The model under review builds one solid part; all positions refer to its coordinate system, in mm. Round coordinates to 2 decimals unless told otherwise and drop trailing zeros. Return JSON: item names as keys, results as strings. Group by question number.
Q1. Consider section A-A (y = 0). Count the separate pieces of the cut face and the enclosed holes in it, and give its area (3 significant figures).
Q2. To check wall thickness, follow line 1 along Y through (x, z) = (0, 0.1) (3 decimals); line 2 along Y through (x, z) = (5.5, 1.3). State the ranges of each line that lie inside material, in increasing order.
Q3. Clearance check with flat-ended pins moving along their axes: pin 1 Ø2 at (y, z) = (1, 1.5) entering from +X; pin 2 Ø1 at (x, z) = (-6, 2.5) entering from +Y; pin 3 Ø2 at (y, z) = (0, 0.5) entering from -X. State where each tip first meets the part, or that it passes through.
from build123d import *

# Parameters (mm, degrees)
SKETCH_1_R      = 16
SKETCH_1_R_2    = 12.5
EXTRUDE_1_DEPTH = 4
EXTRUDE_START   = -2
SKETCH_2_R      = 17
SKETCH_2_R_2    = 16
EXTRUDE_2_DEPTH = 1.1
FILLET_1_R      = 0.1
SKETCH_3_W      = 0.5
SKETCH_3_H      = 1.15


with BuildPart() as part:
    # 草图1 → 凸台-拉伸1 (new body)
    with BuildSketch(Plane.XY):
        Circle(SKETCH_1_R)
        Circle(SKETCH_1_R_2, mode=Mode.SUBTRACT)
    extrude(amount=EXTRUDE_1_DEPTH)

    # 草图2 → 凸台-拉伸2 (add)
    with BuildSketch(Plane.XY.offset(4).offset(EXTRUDE_START)):
        Circle(SKETCH_2_R)
        Circle(SKETCH_2_R_2, mode=Mode.SUBTRACT)
    extrude(amount=EXTRUDE_2_DEPTH)

    # 圆角1
    fillet_1_edges = [part.edges().sort_by_distance(p)[0] for p in [
        (-16, 0, 0),
    ]]
    fillet(fillet_1_edges, radius=FILLET_1_R)

    # 草图3 → 切除-旋转1 (revolve, cut)
    with BuildSketch(Plane(origin=(0, 0, 0), x_dir=(0, 0, -1), z_dir=(1, 0, 0)), mode=Mode.PRIVATE) as cut_revolve_1_sk:
        with Locations((-0.25, 14.25)):
            Rectangle(SKETCH_3_W, SKETCH_3_H)
        with Locations((-2.85, 14.25)):
            Rectangle(SKETCH_3_W, SKETCH_3_H)
    cut_revolve_1 = revolve(cut_revolve_1_sk.sketch.rotate(Axis((0, 0, 0), (0, 0, 1)), 90), axis=Axis((0, 0, 0), (0, 0, 1)), mode=Mode.SUBTRACT)

    # 镜向1: 切除-旋转1 across plane
    add(cut_revolve_1.mirror(Plane(origin=(0, 0, 2), x_dir=(1, 0, 0), z_dir=(0, 0, -1))), mode=Mode.SUBTRACT)


solid = part.part
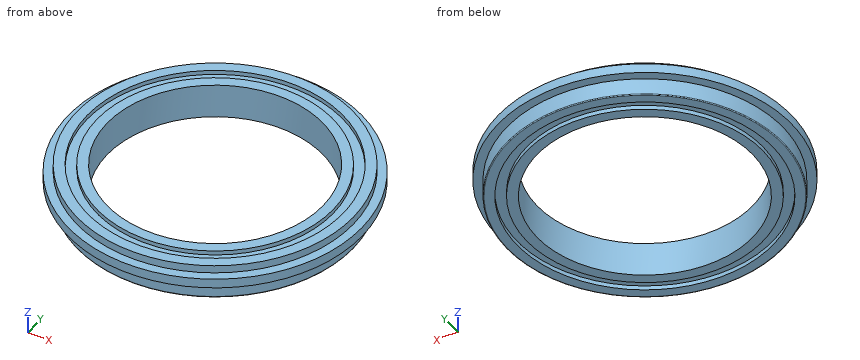
Values:
{
 "1": {"separate pieces": "2", "enclosed holes": "4", "area": "25.6 mm2"},
 "2": {"line 1": "y = -16 to -14.825, -13.675 to -12.5, 12.5 to 13.675, 14.825 to 16", "line 2": "y = -15.02 to -13.77, -12.52 to -11.22, 11.22 to 12.52, 13.77 to 15.02"},
 "3": {"pin 1": "stops at x = 17", "pin 2": "stops at y = 16.09", "pin 3": "stops at x = -16"}
}
